Read the model definition and answer for the solid it produces. Units are mm, in the model's axes. A direction names the side the tool comes from. Give positions to 0.01 mm unless a question says otherwise; leave off trailing zeros. Order: outer loops, then holes, each group sorted by start corner. A loop starts at its lowest first (then second) coordinate and runs counter-clockwise, first axis right, second up. Notation, with made-up numbers: (-38, 55) -> (5, 55) arc R27 cw to (5, 93) -> close; hole circle Ø2 at (-37.5, -26). An arc over 180 degrees is marked (long way). One line per item, written item: value. Start each with the question number.
from build123d import *

# Parameters (mm, degrees)
F0_W     = 48
F0_H     = 48
F1_DEPTH = 3
F2_R     = 2
F3_W     = 44
F3_H     = 44
F3_W_2   = 42.5
F3_H_2   = 42.5
F4_DEPTH = 5
F5_R     = 1


with BuildPart() as f1:
    # F0 (on Top) → F1 (new body)
    with BuildSketch(Plane.XY):
        with Locations((24, -24)):
            Rectangle(F0_W, F0_H)
    extrude(amount=F1_DEPTH)

    # F2
    f2_edges = [f1.edges().sort_by_distance(p)[0] for p in [
        (48, -48, 1.5),
        (0, -48, 1.5),
        (48, 0, 1.5),
        (0, 0, 1.5),
    ]]
    fillet(f2_edges, radius=F2_R)

    # F3 (on face) → F4 (join)
    with BuildSketch(Plane.XY.offset(3)):
        with Locations((24, -24)):
            Rectangle(F3_W, F3_H)
        with Locations((24, -24)):
            Rectangle(F3_W_2, F3_H_2, mode=Mode.SUBTRACT)
    extrude(amount=F4_DEPTH)

    # F5
    f5_edges = [f1.edges().sort_by_distance(p)[0] for p in [
        (46, -2, 5.5),
        (2, -2, 5.5),
        (2, -46, 5.5),
        (46, -46, 5.5),
    ]]
    fillet(f5_edges, radius=F5_R)


solid = f1.part
Item 1: For a pull along Y with two mould halves and no side action, classify faces 1 (the flat face through (24, -46, 5)), 2 (the flat face through (2, -24, 5)), 3 (the flat face through (24, -2.75, 5)) as +Y half, -Y half, draft (parallel to the pull), parting line (faces both ways), or undercut.
Item 2: Find section B-B on y = -39.5. Write down the section's boundary in (x, z), then the cut area to 4 significant figures.
Item 3: Flat-ended cylindrical pins translate along their axes: pin 1 (21 mm diameter, centred on x = 29.5, y = -30.5, fed in from +Z); pin 2 (2.5 mm diameter, centred on y = -28.5, z = 4.5, fed in from +X); pin 3 (4 mm diameter, centred on y = -9, z = 6, fed in from -X). Find the tip coordinate at first contact, or state that the pin passes through.
Item 4: A tool of negligible diameter and unlimited length cuts with its end or side. For faces 4 (the cylindrical face through (0.57, -0.6, 1.52)), 5 (the flat face through (24, -2, 5)), 6 (the flat face through (24, -45.25, 5)), from which of +Z, -Z, +X, -X, +Y, -Y can it reach the whole face along a straight path? Write none if from no direction.
Item 5: Find section C-C on x = 22. Write down the section's boundary in (y, z).
Item 6: Find section A-A on z = 3.75. Write down the section's boundary in (x, y), then the cut area to 3 significant figures.
Item 7: Find the intervals of material crossed by line 1 (X direction, y = -26.5, z = 5.25); line 2 (Y direction, x = 44, z = 6); line 3 (Z direction, x = 25.5, y = -11.5), in increasing order. Write a range as from..to.
Checks:
1. face 1: -Y half
1. face 2: draft
1. face 3: undercut
2. outline: (0, 0) -> (48, 0) -> (48, 3) -> (46, 3) -> (46, 8) -> (45.25, 8) -> (45.25, 3) -> (2.75, 3) -> (2.75, 8) -> (2, 8) -> (2, 3) -> (0, 3) -> close
2. area: 151.5 mm2
3. pin 1: z = 3
3. pin 2: x = 46
3. pin 3: x = 2
4. face 4: +Z, -Z, -X, +Y
4. face 5: +Z, +X, -X, +Y
4. face 6: +Z
5. outline: (-48, 0) -> (0, 0) -> (0, 3) -> (-2, 3) -> (-2, 8) -> (-2.75, 8) -> (-2.75, 3) -> (-45.25, 3) -> (-45.25, 8) -> (-46, 8) -> (-46, 3) -> (-48, 3) -> close
6. outline: (2, -45) arc R1 ccw to (3, -46) -> (45, -46) arc R1 ccw to (46, -45) -> (46, -3) arc R1 ccw to (45, -2) -> (3, -2) arc R1 ccw to (2, -3) -> close; hole (2.75, -45.25) -> (45.25, -45.25) -> (45.25, -2.75) -> (2.75, -2.75) -> close
6. area: 129 mm2
7. line 1: 2..2.75, 45.25..46
7. line 2: -46..-45.25, -2.75..-2
7. line 3: 0..3
